```python
from build123d import *

# Parameters (mm, degrees)
F1_DEPTH  = 13
F2_R      = 16.11
F3_DEPTH  = 16
F3_TAPER  = 8.7
F5_DEPTH  = 1
F6_R      = 3.5
F7_DEPTH  = 60
F9_DEPTH  = 1
F10_DEPTH = 1
F11_DEPTH = 1
F12_DEPTH = 1
F13_R     = 2.625
F14_DEPTH = 15
F15_R     = 3.975
F16_DEPTH = 12.36


# Not quite as in the source:
# - ends of sketch curves that miss each other by under 0.0002 mm in the source are joined


with BuildPart() as f1:
    # F0 (on Top) → F1 (new body)
    with BuildSketch(Plane.XY):
        Polygon((-210, -30), (210, -30), (210, 30), (-210, 30), (-210, 21), (-210, -21), align=None)
    extrude(amount=F1_DEPTH)

    # F2 (on face) → F3 (cut)
    with BuildSketch(Plane.XY.offset(13)):
        with Locations((56, 0)):
            Circle(F2_R)
        with Locations((-59, 0)):
            Circle(F2_R)
    extrude(amount=-F3_DEPTH, taper=F3_TAPER, mode=Mode.SUBTRACT)

    # F4 (on face) → F5 (cut)
    with BuildSketch(Plane(origin=(0, 0, 0), x_dir=(1, 0, 0), z_dir=(0, 0, -1))):
        with BuildLine():
            Line((210, 30), (-184.9498743711, 30))
            ThreePointArc((-184.9498743711, 30), (-181.7082039325, 23.5838015129), (-175, 21))
            Line((-175, 21), (150, 21))
            ThreePointArc((150, 21), (171, 0), (150, -21))
            Line((150, -21), (-175, -21))
            ThreePointArc((-175, -21), (-181.7082039325, -23.5838015129), (-184.9498743711, -30))
            Line((-184.9498743711, -30), (210, -30))
            Line((210, -30), (210, 30))
        make_face()
    extrude(amount=-F5_DEPTH, mode=Mode.SUBTRACT)

    # F6 (on face) → F7 (cut)
    with BuildSketch(Plane(origin=(0, 30, 0), x_dir=(-1, 0, 0), z_dir=(0, 1, 0))):
        with BuildLine():
            ThreePointArc((190, 6.5), (193.5, 3), (197, 6.5))
            Line((197, 6.5), (193.5, 6.5))
            Line((193.5, 6.5), (190, 6.5))
        make_face()
        with BuildLine():
            Line((193.5, 6.5), (197, 6.5))
            ThreePointArc((197, 6.5), (193.5, 10), (190, 6.5))
            Line((190, 6.5), (193.5, 6.5))
        make_face()
        with Locations((33.35, 6.5)):
            Circle(F6_R)
        with Locations((18.2, 6.5)):
            Circle(F6_R)
        with Locations((3.05, 6.5)):
            Circle(F6_R)
        with Locations((-12.1, 6.5)):
            Circle(F6_R)
        with BuildLine():
            ThreePointArc((-30.75, 6.5), (-27.25, 3), (-23.75, 6.5))
            ThreePointArc((-23.75, 6.5), (-27.25, 10), (-30.75, 6.5))
        make_face()
        with Locations((-82.25, 6.5)):
            Circle(F6_R)
        with Locations((-97.4, 6.5)):
            Circle(F6_R)
        with Locations((-112.55, 6.5)):
            Circle(F6_R)
        with Locations((-127.7, 6.5)):
            Circle(F6_R)
        with Locations((-142.85, 6.5)):
            Circle(F6_R)
        with Locations((-158, 6.5)):
            Circle(F6_R)
        with Locations((-173.15, 6.5)):
            Circle(F6_R)
        with Locations((-188.3, 6.5)):
            Circle(F6_R)
    extrude(amount=-F7_DEPTH, mode=Mode.SUBTRACT)

    # F8 (on face) → F9 (cut)
    with BuildSketch(Plane.XY.offset(13)):
        with BuildLine():
            Line((210, 30), (62, 30))
            ThreePointArc((62, 30), (64.6360389693, 23.6360389693), (71, 21))
            Line((71, 21), (210, 21))
            Line((210, 21), (210, 30))
        make_face()
    extrude(amount=-F9_DEPTH, mode=Mode.SUBTRACT)

    # F8 (on face) → F10 (cut)
    with BuildSketch(Plane.XY.offset(13)):
        with BuildLine():
            Line((210, -30), (210, -21))
            Line((210, -21), (71, -21))
            ThreePointArc((71, -21), (64.6360389693, -23.6360389693), (62, -30))
            Line((62, -30), (210, -30))
        make_face()
        with BuildLine():
            ThreePointArc((-44.1668648796, -21), (-50.5308259103, -23.6360389693), (-53.1668648796, -30))
            Line((-53.1668648796, -30), (50, -30))
            Line((50, -30), (61.9996917391, -30))
            Line((61.9996917391, -30), (61.9996917391, -29.9984586954))
            Line((61.9996917391, -29.9984586954), (49.9996917391, -29.9984586954))
            Line((49.9996917391, -29.9984586954), (49.9966373946, -29.8334433813))
            ThreePointArc((49.9966373946, -29.8334433813), (47.3029780787, -23.5774222633), (40.9981786992, -21))
            Line((40.9981786992, -21), (-44.1668648796, -21))
        make_face()
    extrude(amount=-F10_DEPTH, mode=Mode.SUBTRACT)

    # F8 (on face) → F11 (cut)
    with BuildSketch(Plane.XY.offset(13)):
        with BuildLine():
            Line((-74.1668648796, -21), (-210, -21))
            Line((-210, -21), (-210, -30))
            Line((-210, -30), (-65.1668648796, -30))
            ThreePointArc((-65.1668648796, -30), (-67.8029038489, -23.6360389693), (-74.1668648796, -21))
        make_face()
        with BuildLine():
            ThreePointArc((-73.9996917391, 21), (-67.6362756652, 23.6354940592), (-64.9996918711, 29.9984586954))
            Line((-64.9996918711, 29.9984586954), (-64.9996917391, 30))
            Line((-64.9996917391, 30), (-210, 30))
            Line((-210, 30), (-210, 21))
            Line((-210, 21), (-73.9996917391, 21))
        make_face()
    extrude(amount=-F11_DEPTH, mode=Mode.SUBTRACT)

    # F8 (on face) → F12 (cut)
    with BuildSketch(Plane.XY.offset(13)):
        with BuildLine():
            Line((50, 30), (-52.9996917391, 30))
            Line((-52.9996917391, 30), (-52.9996917391, 29.9969173908))
            ThreePointArc((-52.9996917391, 29.9969173908), (-50.3636527698, 23.6329563601), (-43.9996917391, 20.9969173908))
            Line((-43.9996917391, 20.9969173908), (41.0002951444, 20.9997048653))
            ThreePointArc((41.0002951444, 20.9997048653), (47.3640653791, 23.6358481799), (50, 29.9997048604))
            Line((50, 29.9997048604), (50, 30))
        make_face()
    extrude(amount=-F12_DEPTH, mode=Mode.SUBTRACT)

    # F13 (on face) → F14 (cut)
    with BuildSketch(Plane(origin=(-210, 0, 0), x_dir=(0, -1, 0), z_dir=(-1, 0, 0))):
        with Locations((-20, 8)):
            Circle(F13_R)
        with Locations((20, 8)):
            Circle(F13_R)
    extrude(amount=-F14_DEPTH, mode=Mode.SUBTRACT)

    # F15 (on face) → F16 (cut)
    with BuildSketch(Plane.YZ.offset(210)):
        with Locations((0, 6.5)):
            Circle(F15_R)
        with Locations((-15, 6.5)):
            Circle(F15_R)
    extrude(amount=-F16_DEPTH, mode=Mode.SUBTRACT)


solid = f1.part
```
Model file for the job. Use its own axes, mm. A direction names the side the tool comes from. Coordinates: 2 decimals unless noted, no trailing zeros. Loops run counter-clockwise (first coordinate to the right, second up) from the corner with the lowest first, then second, coordinate; pieces in that order, holes last. Notation, with made-up numbers: M 27,-22 L 54,-22 A8 ccw 54,-7 Z; hole C 47,51.5 d9. An arc over 180 degrees is marked long. Use CSV: the item, a comma, the result in double quotes. Start each with the question number.
1. Band-saw the part on A-A, the plane x = 188.3. List the corners of the cut face in (y, z).
2. Two-plate mould, pull along X, no slides. Class faces 1 (the cylindrical face through (116.047, 0.42, 6.654)), 2 (the cylindrical face through (-67.73, -23.71, 12.51)), 3 (the cylindrical face through (64.706, -23.566, 12.507)): pulls with the +X half, pulls with the -X half, needs draft (parallel to the pull), parting line crosses it, or undercut.
3. Tool access for faces 4 (the cylindrical face through (-181.632, 23.515, 0.493)), 5 (the cylindrical face through (64.566, 23.706, 12.507)), 6 (the cylindrical face through (170.995, -0.462, 0.493)), 7 (the flat face through (-2, 26, 12)): list every direction of +Z, -Z, +X, -X, +Y, -Y with a clear straight run to the whole face (end or side of a thin tool).
4. Band-saw the part on B-B, the plane x = 97.4. List the corners of the cut face in (y, z).
5. Band-saw the part on C-C, the plane y = 9. Give the number of separate pieces and of enclosed holes in the cut face, then the cut area to 3 significant figures.
6. Flat gauge pins, fed straight in: pin 1 (0.8 mm diameter, centred on x = 108.5, z = 12.5, fed in from +Y); pin 2 (0.5 mm diameter, centred on y = -20, z = 10, fed in from -X); pin 3 (4.5 mm diameter, centred on x = -3, y = -26, fed in from +Z). Where does each tip first touch, or does it go through?
7. Probe probe 1 along Z at (x, y) = (-193, 15); probe 2 along X at (y, z) = (10, 2.25); probe 3 along X at (y, z) = (-7, 11). List the from-to ranges inside material, lowest first. Write a range as [from, to].
Entries:
1,outline,"M -30,1 L 30,1 L 30,3 L -30,3 Z; M -30,10 L 30,10 L 30,12 L 21,12 L 21,13 L -21,13 L -21,12 L -30,12 Z"
2,face 1,"undercut"
2,face 2,"pulls with the -X half"
2,face 3,"pulls with the +X half"
3,face 4,"-Z, +X, +Y"
3,face 5,"+Z, +X, +Y"
3,face 6,"-Z, +X"
3,face 7,"+Z, +Y"
4,outline,"M -30,1 L -21,1 L -21,0 L 21,0 L 21,1 L 30,1 L 30,3 L -30,3 Z; M -30,10 L 30,10 L 30,12 L 21,12 L 21,13 L -21,13 L -21,12 L -30,12 Z"
5,separate pieces,"3"
5,enclosed holes,"14"
5,area,"4,250 mm2"
6,pin 1,"stops at y = 21"
6,pin 2,"stops at x = -195"
6,pin 3,"stops at z = 12"
7,probe 1,"z = [0, 3.04], [9.96, 13]"
7,probe 2,"x = [-210, -69.45], [-48.55, 45.55], [66.45, 210]"
7,probe 3,"x = [-210, -73.17], [-44.83, 41.83], [70.17, 210]"
